Geometry check sheet. Reference: the model listing, model coordinates, mm. Face numbers are marked on the shaded views. A direction names the side the tool comes from. Round coordinates to 2 decimals unless told otherwise and drop trailing zeros. Write each loop counter-clockwise with the first axis right and the second up, starting at its lowest first coordinate (ties: lowest second). Pieces come first, ordered by that corner, then holes. Notation, with made-up numbers: (19.5, 0.5) - (28.5, 0.5) arc R21 ccw to (28.5, 37.5) - close; hole circle Ø1 at (-13, 11). An arc over 180 degrees is marked (long way). Return JSON: item names as keys, results as strings.
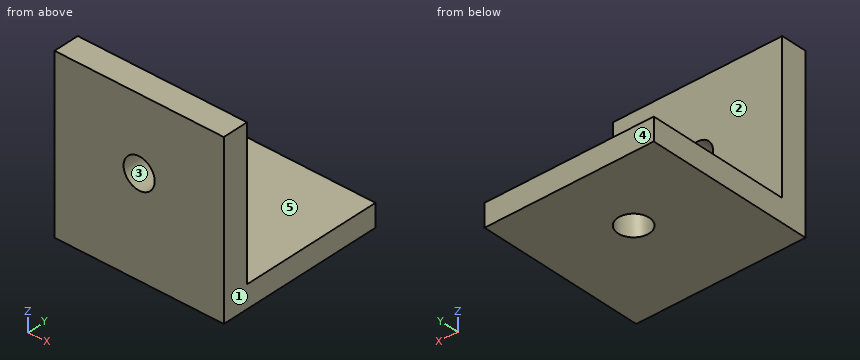
Autodesk Inventor part; units mm, degrees
ref_plane "YZ Plane" through (0, 0, 0) normal (1, 0, 0) x (0, 1, 0)
ref_plane "XZ Plane" through (0, 0, 0) normal (0, 1, 0) x (-1, 0, 0)
ref_plane "XY Plane" through (0, 0, 0) normal (0, 0, 1) x (1, 0, 0)
sketch "Sketch1" plane through (0, 0, 0) normal (0, 1, 0) x (-1, 0, 0)
  line L0 (-13.4529, -30.7592) -> (5.5971, -30.7592)
  line L1 (5.5971, -30.7592) -> (5.5971, -49.8092)
  line L2 (5.5971, -49.8092) -> (-13.4529, -49.8092)
  line L3 (-13.4529, -49.8092) -> (-13.4529, -30.7592)
  line L4 (-13.4529, -30.7592) -> (5.5971, -49.8092) construction
  line L5 (5.5971, -30.7592) -> (-13.4529, -49.8092) construction
  line L6 (-3.9279, -30.7592) -> (-3.9279, -38.8592) construction
  circle A0 centre (-3.9279, -38.8592) radius 1.75
  point P0 (0, 0)
  point P1 (-3.9279, -40.2842)
  dimension "d0" = 19.05
  dimension "d1" = 19.05
  dimension "d8" = 8.1
  dimension "d9" = 3.5
extrude "Extrusion1" add sketch "Sketch1" along normal blind 2.921
sketch "Sketch2" plane through (0, 2.921, 0) normal (0, 1, 0) x (1, 0, 0)
  line L0 (-5.5971, 49.8092) -> (13.4529, 49.8092)
  line L1 (13.4529, 49.8092) -> (13.4529, 47.2692)
  line L2 (13.4529, 47.2692) -> (-5.5971, 47.2692)
  line L3 (-5.5971, 47.2692) -> (-5.5971, 49.8092)
  point P0 (0, 0)
  dimension "d4" = 19.05
  dimension "d5" = 2.54
extrude "Extrusion2" add sketch "Sketch2" along normal blind 16.129
sketch "Sketch3" plane through (13.4529, 0, -49.8092) normal (0, 0, -1) x (-1, 0, 0)
  line L0 (19.05, 0) -> (0, 0) construction
  line L1 (19.05, 0) -> (19.05, 19.05) construction
  line L2 (0, 19.05) -> (19.05, 19.05) construction
  line L3 (0, 0) -> (0, 19.05) construction
  line L4 (0, 19.05) -> (19.05, 19.05) construction
  line L5 (9.525, 19.05) -> (9.525, 10.95) construction
  circle A0 centre (9.525, 10.95) radius 1.75
  point P0 (13.4529, 0)
  dimension "d10" = 8.1
  dimension "d11" = 3.5
extrude "Extrusion3" cut sketch "Sketch3" against normal blind 25.4
(1) Gauge pin test, flat ends, axial feed: pin 1 (8 mm diameter, centred on x = 2, y = 9.5, fed in from +Z); pin 2 (10 mm diameter, centred on y = 5, z = -41.5, fed in from +X); pin 3 (1 mm diameter, centred on x = 4, z = -42, fed in from +Y). Record the tip position at first contact, or that the pin passes through.
Response values:
{"pin 1": "stops at z = -47.27", "pin 2": "stops at x = 13.45", "pin 3": "stops at y = 2.92"}
(2) Release check for a two-part mould opening along Z. For the marked faces 3, 4 and 5 record: pulls with the +Z half, pulls with the -Z half, needs draft (parallel to the pull), parting line crosses it, or undercut.
Response values:
{"face 3": "undercut", "face 4": "needs draft", "face 5": "pulls with the +Z half"}
(3) Section check A-A, the plane y = 10.95. Enter the section's corners in (x, z).
Response values:
{"outline": "(-5.6, -49.81) - (2.18, -49.81) - (2.18, -47.27) - (-5.6, -47.27) - close; (5.68, -49.81) - (13.45, -49.81) - (13.45, -47.27) - (5.68, -47.27) - close"}
(4) Section check D-D, the plane x = 9.75. Enter the section's corners in (y, z).
Response values:
{"outline": "(0, -49.81) - (19.05, -49.81) - (19.05, -47.27) - (2.92, -47.27) - (2.92, -30.76) - (0, -30.76) - close"}
(5) Access from +Z, -Z, +X, -X, +Y, -Y to the whole of each face (thin tool, end or side, straight path). Record for the marked faces 1 and 2.
Response values:
{"face 1": "+Z, -Z, +X, +Y, -Y", "face 2": "+Z, +X, -X, +Y"}
(6) Section check C-C, the plane z = -48. Enter the section's corners in (x, y), plus the area to 3 significant figures.
Response values:
{"outline": "(-5.6, 0) - (13.45, 0) - (13.45, 19.05) - (-5.6, 19.05) - close; hole circle Ø3.5 at (3.93, 10.95)", "area": "353 mm^2"}
(7) Material ranges on line 1 along Y through (x, z) = (11.25, -44.5); line 2 along Z through (x, y) = (8.75, 3), recorded low to high. Write a range as [from, to].
Response values:
{"line 1": "y = [0, 2.92]", "line 2": "z = [-49.81, -47.27]"}
(8) Section check B-B, the plane x = 2.75. Enter the section's corners in (y, z), plus the area to 3 significant figures.
Response values:
{"outline": "(0, -49.81) - (9.66, -49.81) - (9.66, -47.27) - (2.92, -47.27) - (2.92, -40.15) - (0, -40.15) - close; (0, -37.56) - (2.92, -37.56) - (2.92, -30.76) - (0, -30.76) - close; (12.24, -49.81) - (19.05, -49.81) - (19.05, -47.27) - (12.24, -47.27) - close", "area": "82.5 mm^2"}
